Can you work these out from the model? Positions are in its coordinate system, mm. Face numbers are marked on the shaded views. A direction names the side the tool comes from. Round coordinates to 2 decimals unless told otherwise and drop trailing zeros. Order: outer loops, then holes, each group sorted by start corner. A loop starts at its lowest first (then second) coordinate and runs counter-clockwise, first axis right, second up.
Q1. Will these pins go through, and if not, where does the flat tip stop? P1, Ø3, axis at x = 6.5, y = 37, coming from the +Z side; P2, Ø8, axis at x = 3.5, y = -15, coming from the -Z side; P3, Ø5, axis at y = 0.5, z = -7, coming from the +X side; P4, Ø5.5, axis at x = 5, y = -37, coming from the -Z side.
Q2. If we section it at C-C (x = 3.75): Please give me the cut outline in (y, z) (1 decimal), plus the area to 3 significant figures.
Q3. For the marked faces 1, 2, 3, 4 and 5, which set-ups out of +Z, -Z, +X, -X, +Y, -Y let a thin tool reach every point of the face, with its end or its side?
Q4. If we section it at B-B (y = 15): Please give me the cut outline in (x, z).
Q5. If we section it at D-D (x = -3): Please give me the cut outline in (y, z).
Q6. If we section it at A-A (z = 0): Please give me the cut outline in (x, y).
Q7. If I drill on line 1 (Y direction, x = -1.85, z = 0); line 2 (Y direction, x = 5, z = -4.7); line 3 (Z direction, x = -1.7, y = -15), over which ranges is the centre line in solid material (lowest first)?
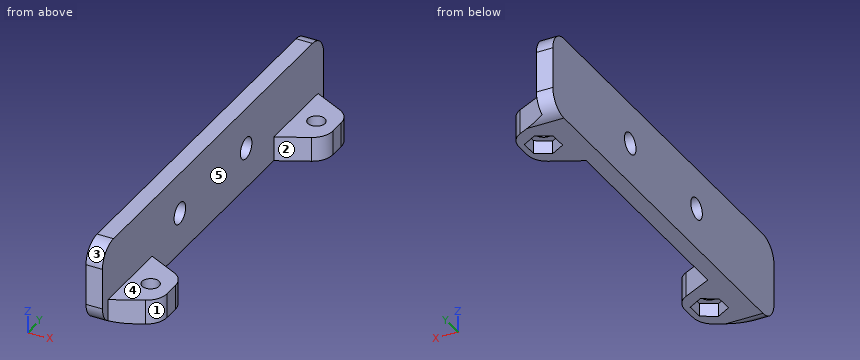
from build123d import *

# Parameters (mm, degrees)
F0_W     = 100
F0_H     = 20
F0_R     = 2.6
F1_DEPTH = 4
F2_R     = 2.1
F3_DEPTH = 6
F4_DEPTH = 3.2
F6_R     = 5


with BuildPart() as f1:
    # F0 (on Right) → F1 (new body)
    with BuildSketch(Plane.YZ):
        Rectangle(F0_W, F0_H)
        with Locations((-15, 0)):
            Circle(F0_R, mode=Mode.SUBTRACT)
        with Locations((15, 0)):
            Circle(F0_R, mode=Mode.SUBTRACT)
    extrude(amount=-F1_DEPTH)

    # F2 (on face) → F3 (join)
    with BuildSketch(Plane(origin=(0, 0, -10), x_dir=(1, 0, 0), z_dir=(0, 0, -1))):
        with BuildLine():
            Line((7.2360679775, 43.8819660113), (0, 47.5))
            Line((0, 47.5), (0, 27.5))
            Line((0, 27.5), (7.2360679775, 31.1180339887))
            ThreePointArc((7.2360679775, 31.1180339887), (9.2532540418, 32.9615143832), (10, 35.5901699437))
            Line((10, 35.5901699437), (10, 39.4098300563))
            ThreePointArc((10, 39.4098300563), (9.2532540418, 42.0384856168), (7.2360679775, 43.8819660113))
        make_face()
        Polygon((5, 41.5991869112), (8.55, 39.5495934556), (8.55, 35.4504065444), (5, 33.4008130888), (1.45, 35.4504065444), (1.45, 39.5495934556), align=None, mode=Mode.SUBTRACT)
        Polygon((8.55, 35.4504065444), (8.55, 39.5495934556), (5, 41.5991869112), (1.45, 39.5495934556), (1.45, 35.4504065444), (5, 33.4008130888), align=None)
        with Locations((5, 37.5)):
            Circle(F2_R, mode=Mode.SUBTRACT)
    extrude(amount=-F3_DEPTH)

    # F2 (on face) → F4 (cut)
    with BuildSketch(Plane(origin=(0, 0, -10), x_dir=(1, 0, 0), z_dir=(0, 0, -1))):
        Polygon((8.55, 35.4504065444), (8.55, 39.5495934556), (5, 41.5991869112), (1.45, 39.5495934556), (1.45, 35.4504065444), (5, 33.4008130888), align=None)
        with Locations((5, 37.5)):
            Circle(F2_R, mode=Mode.SUBTRACT)
    extrude(amount=-F4_DEPTH, mode=Mode.SUBTRACT)

    # F5: F1 across plane


with BuildPart() as f1_1:
    add(f1.part)
    add(f1.part.mirror(Plane.XZ))

    # F6
    f6_edges = [f1_1.edges().sort_by_distance(p)[0] for p in [
        (-2, -50, 10),
        (-2, -50, -10),
        (-2, 50, -10),
        (-2, 50, 10),
    ]]
    fillet(f6_edges, radius=F6_R)


solid = f1_1.part
Solution:
1. P1: stops at z = -4
1. P2: stops at z = -10
1. P3: stops at x = 0
1. P4: stops at z = -6.8
2. outline: (-45.6, -10) arc R5 ccw to (-45, -10) - (-40.9, -10) - (-40.9, -6.8) - (-39.2, -6.8) - (-39.2, -4) - (-45.6, -4) - close; (-35.8, -6.8) - (-34.1, -6.8) - (-34.1, -10) - (-29.4, -10) - (-29.4, -4) - (-35.8, -4) - close; (29.4, -10) - (34.1, -10) - (34.1, -6.8) - (35.8, -6.8) - (35.8, -4) - (29.4, -4) - close; (39.2, -6.8) - (40.9, -6.8) - (40.9, -10) - (45, -10) arc R5 ccw to (45.6, -10) - (45.6, -4) - (39.2, -4) - close
2. area: 133 mm2
3. face 1: +Z, -Z, +X, -Y
3. face 2: +Z, -Z, +X
3. face 3: +Z, +X, -X, -Y
3. face 4: +Z, +X, +Y, -Y
3. face 5: +Z, +X
4. outline: (-4, -10) - (0, -10) - (0, -2.6) - (-4, -2.6) - close; (-4, 2.6) - (0, 2.6) - (0, 10) - (-4, 10) - close
5. outline: (-50, -5) arc R5 ccw to (-45, -10) - (45, -10) arc R5 ccw to (50, -5) - (50, 5) arc R5 ccw to (45, 10) - (-45, 10) arc R5 ccw to (-50, 5) - close; hole circle Ø5.2 at (-15, 0); hole circle Ø5.2 at (15, 0)
6. outline: (-4, -50) - (0, -50) - (0, -17.6) - (-4, -17.6) - close; (-4, -12.4) - (0, -12.4) - (0, 12.4) - (-4, 12.4) - close; (-4, 17.6) - (0, 17.6) - (0, 50) - (-4, 50) - close
7. line 1: y = -50 to -17.6, -12.4 to 12.4, 17.6 to 50
7. line 2: y = -45 to -39.6, -35.4 to -30, 30 to 35.4, 39.6 to 45
7. line 3: z = -10 to -2.6, 2.6 to 10
